Autodesk Inventor part; units mm, degrees
ref_plane "YZ Plane" through (0, 0, 0) normal (1, 0, 0) x (0, 1, 0)
ref_plane "XZ Plane" through (0, 0, 0) normal (0, 1, 0) x (-1, 0, 0)
ref_plane "XY Plane" through (0, 0, 0) normal (0, 0, 1) x (1, 0, 0)
sketch "Esboço1" plane through (0, 0, 0) normal (0, 1, 0) x (-1, 0, 0)
  line L0 (0, 0) -> (-180, 0)
  line L1 (-180, 0) -> (-180, -90)
  line L2 (-180, -90) -> (0, -90)
  line L3 (0, -90) -> (0, 0)
  dimension "d25" = 180
extrude "Extrusão1" add sketch "Esboço1" along normal blind 20
chamfer "Chanfro1" distance 10 angle 45 4 edges at (90, 0, 0) (180, 0, -45) (90, 0, -90) (0, 0, -45)
fillet "Arredondamento1" radius 5 4 edges at (90, 0, -80) (10, 0, -45) (90, 0, -10) (170, 0, -45)
sketch "Esboço4" plane through (0, 20, 0) normal (0, 1, 0) x (1, 0, 0)
  line L0 (0, 90) -> (0, 0)
  line L1 (171.4645, 8.5355) -> (8.5355, 8.5355)
  line L2 (30, 52.75) -> (45.1, 52.75)
  line L3 (45.1, 52.75) -> (45.1, 56.75)
  line L4 (45.1, 56.75) -> (14.1, 56.75)
  line L5 (14.1, 56.75) -> (14.1, 52.75)
  line L6 (14.1, 52.75) -> (30, 52.75)
  line L7 (12.0711, 77.9289) -> (12.0711, 12.0711)
  line L8 (30, 37.25) -> (45.1, 37.25)
  line L9 (45.1, 37.25) -> (45.1, 33.25)
  line L10 (45.1, 33.25) -> (14.1, 33.25)
  line L11 (14.1, 33.25) -> (14.1, 37.25)
  line L12 (14.1, 37.25) -> (30, 37.25)
  dimension "d49" = 15.1
  dimension "d50" = 4
  dimension "d51" = 31
  dimension "d52" = 4
extrude "Extrusão4" add sketch "Esboço4" along normal blind 20
fillet "Arredondamento4" radius 10 4 edges at (45.1, 40, -35.25) (45.1, 40, -54.75) (14.1, 40, -54.75) (14.1, 40, -35.25)
sketch "Esboço6" plane through (14.1, 20, -33.25) normal (0, 0, 1) x (1, 0, 0)
  line L0 (21, 20) -> (10, 20)
  line L1 (31, 0) -> (0, 0)
  line L2 (0, 0) -> (0, 10)
  circle A0 centre (15.5, 10) radius 6.15
  point P0 (-14.1, -20)
  dimension "d54" = 12.3
extrude "Extrusão6" cut sketch "Esboço6" against normal blind 24
properties part number "base"
Can you work these out from the model? Positions are in its coordinate system, mm. A direction names the side the tool comes from. Coordinates: 2 decimals unless noted, no trailing zeros. Order: outer loops, then holes, each group sorted by start corner. A loop starts at its lowest first (then second) coordinate and runs counter-clockwise, first axis right, second up.
1. Thinking about a two-plate mould opening in Z: for faces 3 (the face through (30, 23, -33.25)), 4 (the face through (17.11, 37.15, -54.72)), 5 (the face through (29, 23, -52.75)), 6 (the face through (29, 23, -37.25)), which applies, +Z half, -Z half, draft (parallel to the pull), parting line (faces both ways), or undercut?
2. If we section it at C-C (y = 27.5): Please give me the cut outline in (x, z), then the cut area to 3 significant figures.
3. For faces 1 (the face through (14.1, 25, -55)), 2 (the face through (91.14, 0.39, -10.13)), which set-ups out of +Z, -Z, +X, -X, +Y, -Y let a thin tool reach every point of the face, with its end or its side?
4. If we section it at A-A (z = -42.5): Please give me the cut outline in (x, y), then the cut area to 3 significant figures.
5. If we section it at B-B (x = 29.6): Please give me the cut outline in (y, z), then the cut area to 3 significant figures.
6. If we section it at D-D (x = 50.5): Please give me the cut outline in (y, z).
7. I need wall thicknesses on line 1 (Y direction, x = 29.6, z = -55.7); line 2 (Y direction, x = 54, z = -64); line 3 (X direction, y = 2, z = -12.5). Which ranges of each line are inside material? Lowest first, please.
8. I'm going to push flat-ended pins straight in: pin 1 (14 mm diameter, centred on x = 29.6, y = 30, fed in from -Z); pin 2 (10 mm diameter, centred on y = 17, z = -53.5, fed in from -X); pin 3 (10 mm diameter, centred on x = 109, z = -37, fed in from +Y); pin 4 (3 mm diameter, centred on y = 25.5, z = -36, fed in from -X). Where does each tip first touch, or does it pass through?
Entries:
1. face 3: +Z half
1. face 4: draft
1. face 5: undercut
1. face 6: undercut
2. outline: (14.1, -56.75) - (23.98, -56.75) - (23.98, -52.75) - (14.1, -52.75) - close; (14.1, -37.25) - (23.98, -37.25) - (23.98, -33.25) - (14.1, -33.25) - close; (35.22, -56.75) - (45.1, -56.75) - (45.1, -52.75) - (35.22, -52.75) - close; (35.22, -37.25) - (45.1, -37.25) - (45.1, -33.25) - (35.22, -33.25) - close
2. area: 158 mm2
3. face 1: +Z, -Z, -X, +Y
3. face 2: +Z, +X, -X, -Y
4. outline: (0, 10) - (8.54, 1.46) arc R5 ccw to (12.07, 0) - (167.93, 0) arc R5 ccw to (171.46, 1.46) - (180, 10) - (180, 20) - (0, 20) - close
4. area: 3,500 mm2
5. outline: (0, -77.93) arc R5 ccw to (1.46, -81.46) - (10, -90) - (20, -90) - (20, -56.75) - (23.85, -56.75) - (23.85, -52.75) - (20, -52.75) - (20, -37.25) - (23.85, -37.25) - (23.85, -33.25) - (20, -33.25) - (20, 0) - (10, 0) - (1.46, -8.54) arc R5 ccw to (0, -12.07) - close; (36.15, -56.75) - (40, -56.75) - (40, -52.75) - (36.15, -52.75) - close; (36.15, -37.25) - (40, -37.25) - (40, -33.25) - (36.15, -33.25) - close
5. area: 1,760 mm2
6. outline: (0, -77.93) arc R5 ccw to (1.46, -81.46) - (10, -90) - (20, -90) - (20, 0) - (10, 0) - (1.46, -8.54) arc R5 ccw to (0, -12.07) - close
7. line 1: y = 0 to 23.85, 36.15 to 40
7. line 2: y = 0 to 20
7. line 3: x = 8 to 172
8. pin 1: stops at z = -56.75
8. pin 2: stops at x = 0
8. pin 3: stops at y = 20
8. pin 4: stops at x = 14.1
